Part print with two shaded views. Sizes in mm from the minimum x, y, z corner. A direction names the side the tool comes from. Give positions to 0.01 mm unless a question says otherwise; leave off trailing zeros. Write each loop counter-clockwise with the first axis right and the second up, starting at its lowest first coordinate (ties: lowest second). Pieces come first, ordered by that corner, then holes. Notation, with made-up numbers: (-11.5, 2.25) -> (22.5, 2.25) arc R14 ccw to (22.5, 24.25) -> close; hole circle Ø7 at (14, -35). An arc over 180 degrees is marked (long way). Answer as a JSON object with one key per item and string values.
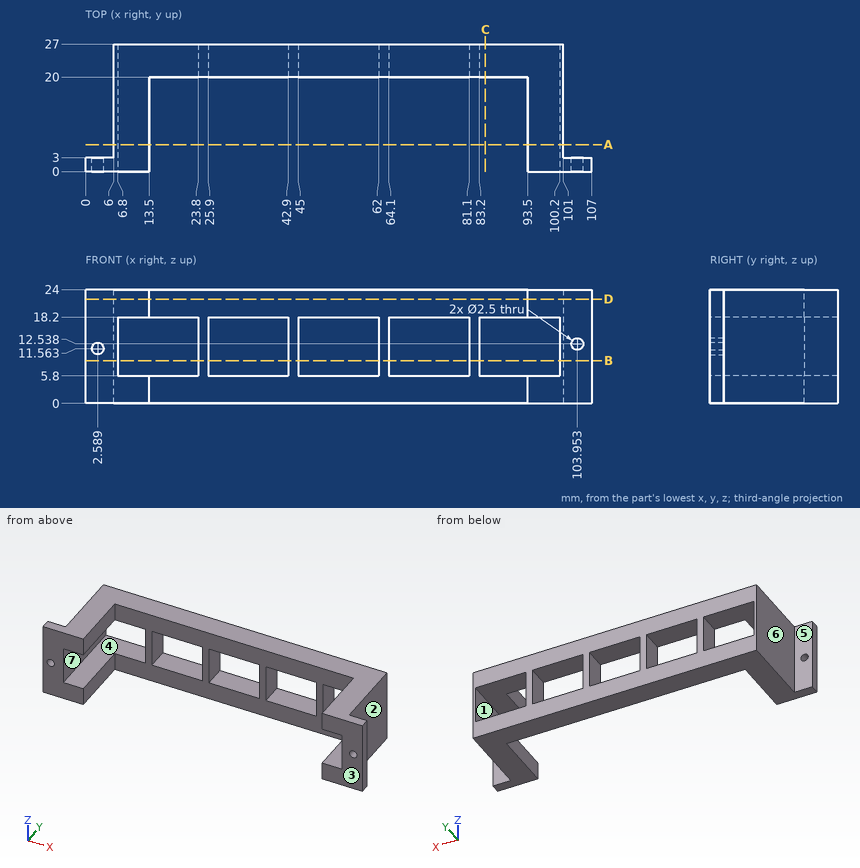
1) Wall check: probe 1 along X at (y, z) = (23.25, 17.5); probe 2 along X at (y, z) = (18.75, 14.75); probe 3 along X at (y, z) = (11.75, 22.75). Give the ranges that are in metal, low to high.
Model answer:
{"probe 1": "x = 6 to 6.8, 23.8 to 25.9, 42.9 to 45, 62 to 64.1, 81.1 to 83.2, 100.2 to 101", "probe 2": "x = 6 to 6.8, 100.2 to 101", "probe 3": "x = 6 to 13.5, 93.5 to 101"}
2) Slice it at C-C (x = 84.5). List the corners of the cut face in (y, z), then the cut area to 3 significant figures.
Model answer:
{"outline": "(20, 0) -> (27, 0) -> (27, 5.8) -> (20, 5.8) -> close; (20, 18.2) -> (27, 18.2) -> (27, 24) -> (20, 24) -> close", "area": "81.2 mm2"}
3) 3-axis set-ups, long thin cutter, end or side, ignore diameter. For the marked faces 1, 2 and 3: which of +Z, -Z, +X, -X, +Y, -Y reach the whole face in a straight line?
Model answer:
{"face 1": "+Y, -Y", "face 2": "+Z, -Z, +X, +Y", "face 3": "+Z, -Z, +X, -X, -Y"}
4) Mould opens along X. For the marked faces 4, 5, 6 and 7 say: released by +X, released by -X, zero draft, split by the parting line, or undercut.
Model answer:
{"face 4": "undercut", "face 5": "zero draft", "face 6": "released by -X", "face 7": "undercut"}
5) Slice it at A-A (y = 5.75). List the corners of the cut face in (x, z).
Model answer:
{"outline": "(6, 0) -> (13.5, 0) -> (13.5, 5.8) -> (6.8, 5.8) -> (6.8, 18.2) -> (13.5, 18.2) -> (13.5, 24) -> (6, 24) -> close; (93.5, 0) -> (101, 0) -> (101, 24) -> (93.5, 24) -> (93.5, 18.2) -> (100.2, 18.2) -> (100.2, 5.8) -> (93.5, 5.8) -> close"}
6) Slice it at D-D (z = 22). List the corners of the cut face in (x, y).
Model answer:
{"outline": "(0, 0) -> (13.5, 0) -> (13.5, 20) -> (93.5, 20) -> (93.5, 0) -> (107, 0) -> (107, 3) -> (101, 3) -> (101, 27) -> (6, 27) -> (6, 3) -> (0, 3) -> close"}
7) Pin check, flat tips, straight feed: pin 1 (3 mm diameter, centred on y = 13.5, z = 4, fed in from -X); pin 2 (3.5 mm diameter, centred on y = 23.5, z = 9, fed in from +X); pin 3 (3 mm diameter, centred on x = 2.59, z = 11.56, fed in from +Y). Stop position of each tip, or through.
Model answer:
{"pin 1": "stops at x = 6", "pin 2": "stops at x = 101", "pin 3": "stops at y = 3"}
8) Slice it at B-B (z = 9). List the corners of the cut face in (x, y), then the cut area to 3 significant figures.
Model answer:
{"outline": "(0, 0) -> (6.8, 0) -> (6.8, 27) -> (6, 27) -> (6, 3) -> (0, 3) -> close; (23.8, 20) -> (25.9, 20) -> (25.9, 27) -> (23.8, 27) -> close; (42.9, 20) -> (45, 20) -> (45, 27) -> (42.9, 27) -> close; (62, 20) -> (64.1, 20) -> (64.1, 27) -> (62, 27) -> close; (81.1, 20) -> (83.2, 20) -> (83.2, 27) -> (81.1, 27) -> close; (100.2, 0) -> (107, 0) -> (107, 3) -> (101, 3) -> (101, 27) -> (100.2, 27) -> close", "area": "138 mm2"}
